from build123d import *

# Parameters (mm, degrees)
F1_DEPTH = 60
F3_D     = 41
F3_DEPTH = 50
F3_TIP   = 12.3176426901
F6_DEPTH = 60


with BuildPart() as f1:
    # F0 (on Top) → F1 (new body)
    with BuildSketch(Plane.XY):
        Polygon((130, 60), (0, 60), (0, 30), (0, 0), (70, 0), align=None)
    extrude(amount=F1_DEPTH)

    # F3
    with Locations(Plane(origin=(0, 0, 0), x_dir=(0, -1, 0), z_dir=(-1, 0, 0))):
        with Locations((-30, 30)):
            Hole(F3_D / 2, depth=F3_DEPTH)
            with Locations((0, 0, -(F3_DEPTH + F3_TIP / 2))):  # 118° drill point
                Cone(0, F3_D / 2, F3_TIP, mode=Mode.SUBTRACT)

    # F4: F1 across face


with BuildPart() as f1_1:
    add(f1.part)
    add(f1.part.mirror(Plane(origin=(100, 30, 30), x_dir=(0.7071067812, 0.7071067812, 0), z_dir=(0.7071067812, -0.7071067812, 0))))

    # F5 (on Top) → F6 (join)
    with BuildSketch(Plane.XY):
        Polygon((70.0001195073, 0), (0, 0), (70.0001195073, -69.9999108911), align=None)
    extrude(amount=F6_DEPTH)


solid = f1_1.part
The listing builds one solid part. Answer for the finished solid, in the listing's coordinates (mm). A direction names the side the tool comes from. Round coordinates to 2 decimals unless told otherwise and drop trailing zeros. Order: outer loops, then holes, each group sorted by start corner. A loop starts at its lowest first (then second) coordinate and runs counter-clockwise, first axis right, second up. Notation, with made-up numbers: M -33.75,80.25 L -25.75,80.25 A34 cw -25.75,118.25 Z; hole C -11,41 d8. An arc over 180 degrees is marked long. Answer in a Markdown table with one row per item. Add a question column.
1) Consider line 1 along Z through (x, y) = (33, 30); line 2 along X through (y, z) = (-50, 30); line 3 along Z through (x, y) = (40.5, 20). Determine where each line is inside the solid, lowest interval first. Write a range as from..to.
2) The part is cut by section B-B on y = -5. Determine the outline of the cut face in (x, z).
3) Determine the mould class of faces 1 (the face through (66, 60, 30)), 2 (the face through (66, -6, 60)), 3 (the face through (96.604, -9.822, 31.069)) for opening direction Z: pulls with the +Z half, pulls with the -Z half, needs draft (parallel to the pull), parting line crosses it, or undercut.
4) The part is cut by section A-A on y = -28. Determine the outline of the cut face in (x, z).
5) Flat-ended cylindrical pins translate along their axes: pin 1 Ø4 at (x, z) = (51.5, 48) entering from -Y; pin 2 Ø10 at (y, z) = (-10.5, 48) entering from -X; pin 3 Ø5 at (x, z) = (19, 15.5) entering from -Y. Find the tip coordinate at first contact, or state that the pin passes through.
6) Which of the six approach directions +Z, -Z, +X, -X, +Y, -Y give full straight-line access (tool end or side, diameter ignored) to faces 4 (the face through (25.35, 49.553, 36.158)), 5 (the face through (118.937, -44.65, 22.148)), 6 (the face through (0, 24, 50))?
Findings below:
| question | item | result |
|---|---|---|
| 1 | line 1 | z = 0..9.5, 50.5..60 |
| 1 | line 2 | x = 50..79.5, 120.5..130 |
| 1 | line 3 | z = 0..12.1, 47.9..60 |
| 2 | outline | M 5,0 L 130,0 L 130,60 L 5,60 Z |
| 3 | face 1 | needs draft |
| 3 | face 2 | pulls with the +Z half |
| 3 | face 3 | undercut |
| 4 | outline | M 28,0 L 130,0 L 130,60 L 28,60 Z; hole C 100,30 d41 |
| 5 | pin 1 | stops at y = -53.5 |
| 5 | pin 2 | stops at x = 5.5 |
| 5 | pin 3 | stops at y = -21.5 |
| 6 | face 4 | -X |
| 6 | face 5 | -Y |
| 6 | face 6 | +Z, -Z, -X, +Y, -Y |
